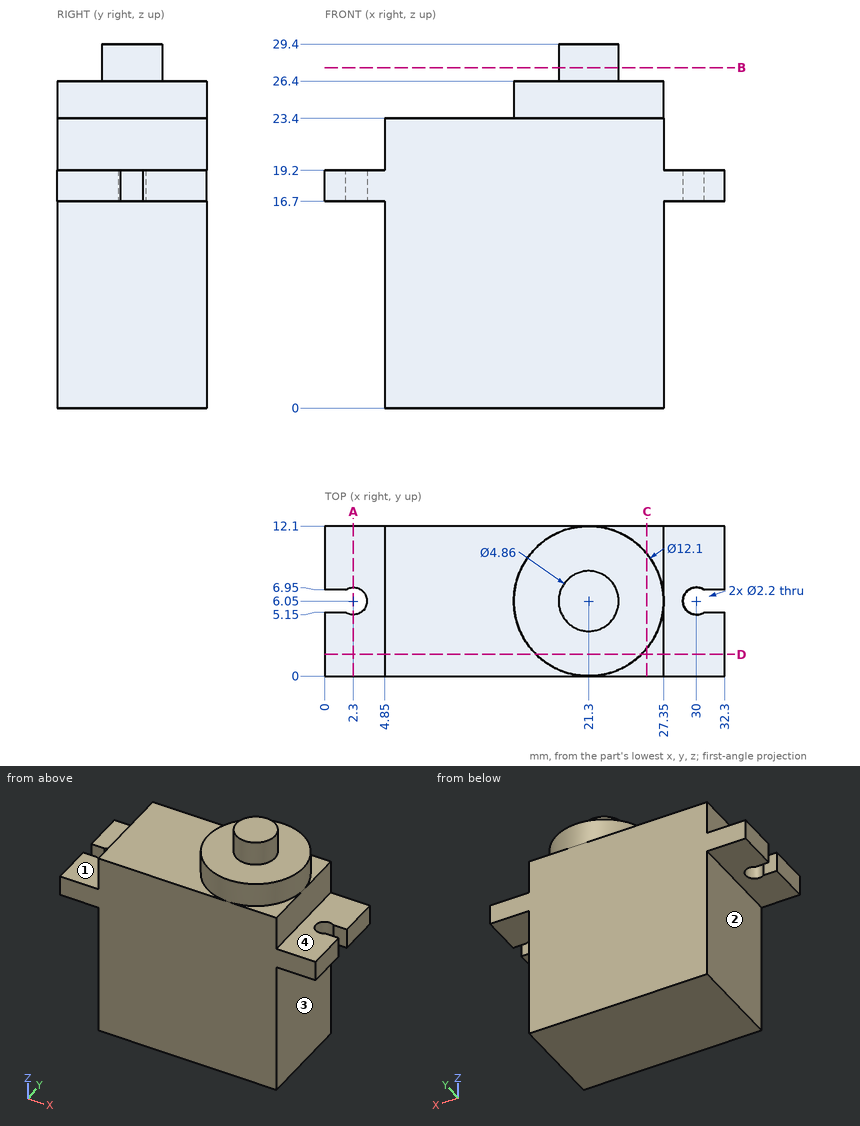
Design review of the part shown in the three views and the two pictorial views. Dimensions are in mm from the part's minimum x, y and z. A direction names the side the tool comes from. Round coordinates to 2 decimals unless told otherwise and drop trailing zeros. Write each loop counter-clockwise with the first axis right and the second up, starting at its lowest first coordinate (ties: lowest second). Pieces come first, ordered by that corner, then holes.
Item 1: We need section A-A on x = 2.3. Write out the cut boundary in (y, z).
Item 2: For probe 1 along Y at (x, z) = (2.3, 17.75); probe 2 along X at (y, z) = (3, 8); probe 3 along X at (y, z) = (6.05, 18.65), list the stretches that pass through material, from the lowest coordinate up.
Item 3: We need section B-B on z = 27.5. Write out the cut boundary in (x, y), and give its area (3 significant figures).
Item 4: For the marked faces 1, 2, 3 and 4, list the 3-axis set-ups (+Z, -Z, +X, -X, +Y, -Y) from which the entire face can be reached by the end or side of a thin tool; tool diameter is ignored.
Item 5: We need section D-D on y = 1.75. Write out the cut boundary in (x, z).
Item 6: We need section C-C on x = 26. Write out the cut boundary in (y, z).
Item 7: Clearance check with flat-ended pins moving along their axes: pin 1 Ø3.5 at (y, z) = (5.5, 9.5) entering from -X; pin 2 Ø4 at (y, z) = (9.5, 8) entering from +X; pin 3 Ø2.5 at (x, y) = (31, 6) entering from +Z. State where each tip first meets the part, or that it passes through.
Returned:
1. outline: (0, 16.7) - (4.95, 16.7) - (4.95, 19.2) - (0, 19.2) - close; (7.15, 16.7) - (12.1, 16.7) - (12.1, 19.2) - (7.15, 19.2) - close
2. probe 1: y = 0 to 4.95, 7.15 to 12.1
2. probe 2: x = 4.85 to 27.35
2. probe 3: x = 3.4 to 28.9
3. outline: circle Ø4.86 at (21.3, 6.05)
3. area: 18.6 mm2
4. face 1: +Z, -X, +Y, -Y
4. face 2: -Z, -X, +Y, -Y
4. face 3: -Z, +X, +Y, -Y
4. face 4: +Z, +X, +Y, -Y
5. outline: (0, 16.7) - (4.85, 16.7) - (4.85, 0) - (27.35, 0) - (27.35, 16.7) - (32.3, 16.7) - (32.3, 19.2) - (27.35, 19.2) - (27.35, 23.4) - (25.56, 23.4) - (25.56, 26.4) - (17.04, 26.4) - (17.04, 23.4) - (4.85, 23.4) - (4.85, 19.2) - (0, 19.2) - close
6. outline: (0, 0) - (12.1, 0) - (12.1, 23.4) - (9.86, 23.4) - (9.86, 26.4) - (2.24, 26.4) - (2.24, 23.4) - (0, 23.4) - close
7. pin 1: stops at x = 4.85
7. pin 2: stops at x = 27.35
7. pin 3: stops at z = 19.2
